```python
from build123d import *

# Parameters (mm, degrees)
F0_R     = 6.4
F1_DEPTH = 4.7
F2_R     = 3.2
F3_DEPTH = 25
F4_SIZE  = 0.5
F5_SIZE  = 0.5


with BuildPart() as f1:
    # F0 (on Top) → F1 (new body)
    with BuildSketch(Plane.XY):
        Circle(F0_R)
    extrude(amount=F1_DEPTH)

    # F2 (on face) → F3 (cut)
    with BuildSketch(Plane.XY.offset(4.7)):
        Circle(F2_R)
    extrude(amount=-F3_DEPTH, mode=Mode.SUBTRACT)

    # F4
    f4_edges = [f1.edges().sort_by_distance(p)[0] for p in [
        (-6.4, 0, 4.7),
        (-3.2, 0, 4.7),
    ]]
    chamfer(f4_edges, length=F4_SIZE)

    # F5
    f5_edges = [f1.edges().sort_by_distance(p)[0] for p in [
        (-6.4, 0, 0),
    ]]
    chamfer(f5_edges, length=F5_SIZE)


solid = f1.part
```
Work out the finished part from the listing and answer in its coordinate system (mm). Coordinates: 2 decimals unless noted, no trailing zeros. Order: outer loops, then holes, each group sorted by start corner. A loop starts at its lowest first (then second) coordinate and runs counter-clockwise, first axis right, second up. Notation, with made-up numbers: M 18.25,2 L 54.25,2 A24 cw 54.25,26 Z; hole C 53.5,44 d8. An arc over 180 degrees is marked long. Use CSV: the item, a comma, the result in double quotes.
1) Section C-C on z = 4.35 is taken. Write down the section's boundary in (x, y).
Worked out:
outline,"C 0,0 d12.5; hole C 0,0 d6.7"
2) Determine the mould class of faces 1 (the face through (-5.08, -3.89, 2.32)), 2 (the face through (3, 3, 4.7)), 3 (the face through (-2.539, -1.947, 2.129)) for opening direction X: released by +X, released by -X, zero draft, split by the parting line, or undercut.
Worked out:
face 1,"split by the parting line"
face 2,"zero draft"
face 3,"undercut"
3) Consider line 1 (Y direction, x = 0, z = 1.9); line 2 (X direction, y = -2.5, z = 2.35); line 3 (X direction, y = 1.5, z = 0.4). Determine where each line is inside the solid, lowest interval first. Write a range as [from, to].
Worked out:
line 1,"y = [-6.4, -3.2], [3.2, 6.4]"
line 2,"x = [-5.89, -2], [2, 5.89]"
line 3,"x = [-6.12, -2.83], [2.83, 6.12]"
4) Section B-B on z = 3.45 is taken. Write down the section's boundary in (x, y).
Worked out:
outline,"C 0,0 d12.8; hole C 0,0 d6.4"
5) Section A-A on x = 0 is taken. Write down the section's boundary in (y, z), plus the area to 3 significant figures.
Worked out:
outline,"M -6.4,0.5 L -5.9,0 L -3.2,0 L -3.2,4.2 L -3.7,4.7 L -5.9,4.7 L -6.4,4.2 Z; M 3.2,0 L 5.9,0 L 6.4,0.5 L 6.4,4.2 L 5.9,4.7 L 3.7,4.7 L 3.2,4.2 Z"
area,"29.3 mm^2"
